Could you check a few things on this model? Use its own coordinates, in mm. A direction names the side the tool comes from. Give positions to 0.01 mm unless a question says otherwise; leave off trailing zeros. Write each loop counter-clockwise with the first axis right and the second up, starting at its lowest first coordinate (ties: lowest second). Pieces come first, ordered by that corner, then holes. Notation, with made-up numbers: M 51.5,61.25 L 63.5,61.25 A23 cw 63.5,85.25 Z; hole C -17,-6 d7. An arc over 180 degrees is marked long. Use one line per item in the form item = value.
from build123d import *

# Parameters (mm, degrees)
SKETCH1_W           = 57.15
SKETCH1_H           = 29.21
BOSS_EXTRUDE1_DEPTH = 30.48
SHELL1_T            = -2.54
SKETCH2_W           = 10.668
SKETCH2_H           = 12.954
CUT_EXTRUDE1_DEPTH  = 2.54
BOSS_EXTRUDE2_DEPTH = 6.35
CUT_EXTRUDE2_REACH  = 68.396
SKETCH4_W           = 9.398
SKETCH4_H           = 7.112
SKETCH6_W           = 33.02
SKETCH6_H           = 3.81
BOSS_EXTRUDE3_DEPTH = 30.48
SKETCH7_W           = 27.94
SKETCH7_H           = 3.81
CUT_EXTRUDE3_DEPTH  = 27.94
FILLET1_R           = 2.54
FILLET2_R           = 1.27
SKETCH8_R           = 3.81
CUT_EXTRUDE4_DEPTH  = 2.54


with BuildPart() as part:
    # Sketch1 → Boss-Extrude1 (new body)
    with BuildSketch(Plane(origin=(0, 0, 0), x_dir=(1, 0, 0), z_dir=(0, 1, 0))):
        Rectangle(SKETCH1_W, SKETCH1_H)
    extrude(amount=BOSS_EXTRUDE1_DEPTH)

    # Shell1
    shell1_openings = [part.faces().sort_by_distance(p)[0] for p in [
        (0, 30.48, 0),
    ]]
    offset(amount=SHELL1_T, openings=shell1_openings, kind=Kind.INTERSECTION)

    # Sketch2 → Cut-Extrude1 (cut)
    with BuildSketch(Plane.XZ):
        with Locations((18.796, 0)):
            Rectangle(SKETCH2_W, SKETCH2_H)
    extrude(amount=-CUT_EXTRUDE1_DEPTH, mode=Mode.SUBTRACT)

    # Sketch3 → Boss-Extrude2 (add)
    with BuildSketch(Plane(origin=(0, 30.48, 0), x_dir=(1, 0, 0), z_dir=(0, 1, 0))):
        with BuildLine():
            Line((-26.035, 12.065), (-26.035, 6.858))
            Line((-26.035, 6.858), (-21.6408, 6.858))
            ThreePointArc((-21.6408, 6.858), (-20.257840557, 7.430840557), (-19.685, 8.8138))
            Line((-19.685, 8.8138), (-19.685, 12.065))
            Line((-19.685, 12.065), (-26.035, 12.065))
        make_face()
        with BuildLine():
            Line((-19.685, -12.065), (-19.685, -8.8138))
            ThreePointArc((-19.685, -8.8138), (-20.257840557, -7.430840557), (-21.6408, -6.858))
            Line((-21.6408, -6.858), (-26.035, -6.858))
            Line((-26.035, -6.858), (-26.035, -12.065))
            Line((-26.035, -12.065), (-19.685, -12.065))
        make_face()
        with BuildLine():
            Line((26.035, 12.065), (22.8092, 12.065))
            Line((22.8092, 12.065), (22.8092, 9.0805))
            ThreePointArc((22.8092, 9.0805), (23.181174388, 8.182474388), (24.0792, 7.8105))
            Line((24.0792, 7.8105), (26.035, 7.8105))
            Line((26.035, 7.8105), (26.035, 12.065))
        make_face()
        with BuildLine():
            Line((26.035, -7.8105), (26.035, -12.065))
            Line((26.035, -12.065), (22.8092, -12.065))
            Line((22.8092, -12.065), (22.8092, -9.0805))
            ThreePointArc((22.8092, -9.0805), (23.181174388, -8.182474388), (24.0792, -7.8105))
            Line((24.0792, -7.8105), (26.035, -7.8105))
        make_face()
    extrude(amount=-BOSS_EXTRUDE2_DEPTH)

    # Cut-Extrude2: up to this face of the body (flat: up to its plane)
    cut_extrude2_end = Plane(part.part.faces().sort_by_distance((28.575, 15.24, 0))[0])
    # Sketch4 → Cut-Extrude2 (cut, up to the picked face)
    with BuildSketch(Plane.ZY.offset(28.575), mode=Mode.PRIVATE) as cut_extrude2_sk1:
        with Locations((0, 30.48)):
            Rectangle(SKETCH4_W, SKETCH4_H)
    cut_extrude2_tool1 = split(extrude(cut_extrude2_sk1.sketch, amount=-CUT_EXTRUDE2_REACH, mode=Mode.PRIVATE), bisect_by=cut_extrude2_end, keep=Keep.BOTH, mode=Mode.PRIVATE)
    add(cut_extrude2_tool1.solids().sort_by(Axis((-28.575, 30.48, 0), (1, 0, 0)))[0], mode=Mode.SUBTRACT)

    # Sketch6 → Boss-Extrude3 (add)
    with BuildSketch(Plane(origin=(0, 30.48, 0), x_dir=(1, 0, 0), z_dir=(0, 1, 0))):
        with Locations((0, -16.51)):
            Rectangle(SKETCH6_W, SKETCH6_H)
    extrude(amount=-BOSS_EXTRUDE3_DEPTH)

    # Sketch7 → Cut-Extrude3 (cut)
    with BuildSketch(Plane(origin=(0, 30.48, 0), x_dir=(1, 0, 0), z_dir=(0, 1, 0))):
        with Locations((0, -13.97)):
            Rectangle(SKETCH7_W, SKETCH7_H)
    extrude(amount=-CUT_EXTRUDE3_DEPTH, mode=Mode.SUBTRACT)

    # Fillet1
    fillet1_edges = [part.edges().sort_by_distance(p)[0] for p in [
        (16.51, 15.24, 14.605),
        (-16.51, 15.24, 14.605),
    ]]
    fillet(fillet1_edges, radius=FILLET1_R)

    # Fillet2
    fillet2_edges = [part.edges().sort_by_distance(p)[0] for p in [
        (28.575, 15.24, 14.605),
        (-28.575, 15.24, 14.605),
        (-28.575, 15.24, -14.605),
        (28.575, 15.24, -14.605),
    ]]
    fillet(fillet2_edges, radius=FILLET2_R)

    # Sketch8 → Cut-Extrude4 (cut)
    with BuildSketch(Plane(origin=(0, 0, -14.605), x_dir=(-1, 0, 0), z_dir=(0, 0, -1))):
        with Locations((-9.68413116, 16.745112741)):
            Circle(SKETCH8_R)
    extrude(amount=-CUT_EXTRUDE4_DEPTH, mode=Mode.SUBTRACT)


solid = part.part
1) I want a section at C-C, the plane y = 5.5. Please give me the cut outline in (x, z) (3 decimals), plus the area to 3 significant figures.
Checked values:
outline = M -28.575,-13.335 A1.27 ccw -27.305,-14.605 L 27.305,-14.605 A1.27 ccw 28.575,-13.335 L 28.575,13.335 A1.27 ccw 27.305,14.605 L 19.05,14.605 A2.54 cw 16.51,17.145 L 16.51,18.415 L -16.51,18.415 L -16.51,17.145 A2.54 cw -19.05,14.605 L -27.305,14.605 A1.27 ccw -28.575,13.335 Z; hole M -26.035,-12.065 L 26.035,-12.065 L 26.035,12.065 L 13.97,12.065 L 13.97,15.875 L -13.97,15.875 L -13.97,12.065 L -26.035,12.065 Z
area = 434 mm2
2) For faces 5 (the flat face through (-23, 15, 14.605)), 6 (the cylindrical face through (23.171, 27.349, -8.192)), 7 (the flat face through (19, 1, -6.477)), 8 (the flat face through (-27, 26.924, 0)), 9 (the flat face through (-23, 24.13, 9)), which set-ups out of +Z, -Z, +X, -X, +Y, -Y let a thin tool reach every point of the face, with its end or its side?
Checked values:
face_5 = +Z, -X, +Y, -Y
face_6 = +Y
face_7 = +Y, -Y
face_8 = +X, -X, +Y
face_9 = none
3) For pin 1 Ø8.5 at (x, z) = (11, 6.5) entering from +Y; pin 2 Ø5 at (x, y) = (-24.5, 27) entering from +Z (3 decimals); pin 3 Ø0.8 at (x, y) = (18, 1) entering from +Z, each with a flat end and sliding along its axis, tell me the tip position at first contact or that it passes through.
Checked values:
pin_1 = 2.54
pin_2 = 14.605
pin_3 = 15.06
4) I want a section at A-A, the plane z = -3.5. Please give me the cut outline in (x, y) (3 decimals), plus the area to 3 significant figures.
Checked values:
outline = M -28.575,0 L 13.462,0 L 13.462,2.54 L -26.035,2.54 L -26.035,26.924 L -28.575,26.924 Z; M 24.13,0 L 28.575,0 L 28.575,26.924 L 26.035,26.924 L 26.035,2.54 L 24.13,2.54 Z
area = 242 mm2
5) If I drill on L1, parallel to Z at x = 1, y = 25 (3 decimals); L2, parallel to X at y = 2.5, z = -0.5 (3 decimals); L3, parallel to X at y = 12, z = 12 (3 decimals), over which ranges is the centre line in solid material (lowest first)?
Checked values:
L1 = -14.605 to -12.065, 15.875 to 18.415
L2 = -28.575 to 13.462, 24.13 to 28.575
L3 = -28.575 to -26.035, 26.035 to 28.575
6) I want a section at B-B, the plane x = -1.5. Please give me the cut outline in (y, z) (3 decimals), plus the area to 3 significant figures.
Checked values:
outline = M 0,-14.605 L 30.48,-14.605 L 30.48,-12.065 L 2.54,-12.065 L 2.54,15.875 L 30.48,15.875 L 30.48,18.415 L 0,18.415 Z
area = 226 mm2
7) I want a section at D-D, the plane z = 10. Please give me the cut outline in (x, y) (3 decimals).
Checked values:
outline = M -28.575,0 L 28.575,0 L 28.575,30.48 L 22.809,30.48 L 22.809,24.13 L 26.035,24.13 L 26.035,2.54 L -26.035,2.54 L -26.035,24.13 L -19.685,24.13 L -19.685,30.48 L -28.575,30.48 Z
8) Thinking about a two-plate mould opening in X: for faces 1 (the flat face through (-23, 24.13, -9)), 2 (the flat face through (-28.575, 15, 0)), 3 (the flat face through (23, 15, 14.605)), 4 (the flat face through (0, 16, -12.065)), which applies, released by +X, released by -X, zero draft, split by the parting line, or undercut?
Checked values:
face_1 = undercut
face_2 = released by -X
face_3 = zero draft
face_4 = undercut
